Check sheet for the drawn part. Datum: minimum x, y, z corner. Units: mm. A direction names the side the tool comes from. Round coordinates to 2 decimals unless told otherwise and drop trailing zeros. Write each loop counter-clockwise with the first axis right and the second up, starting at its lowest first coordinate (ties: lowest second). Pieces come first, ordered by that corner, then holes. Notation, with made-up numbers: (27.5, -34.5) - (53.5, -34.5) arc R12 ccw to (53.5, -27.5) - close; hole circle Ø5 at (35, 13.5). An arc over 180 degrees is marked (long way). Answer as a JSON object with one key per item and string values.
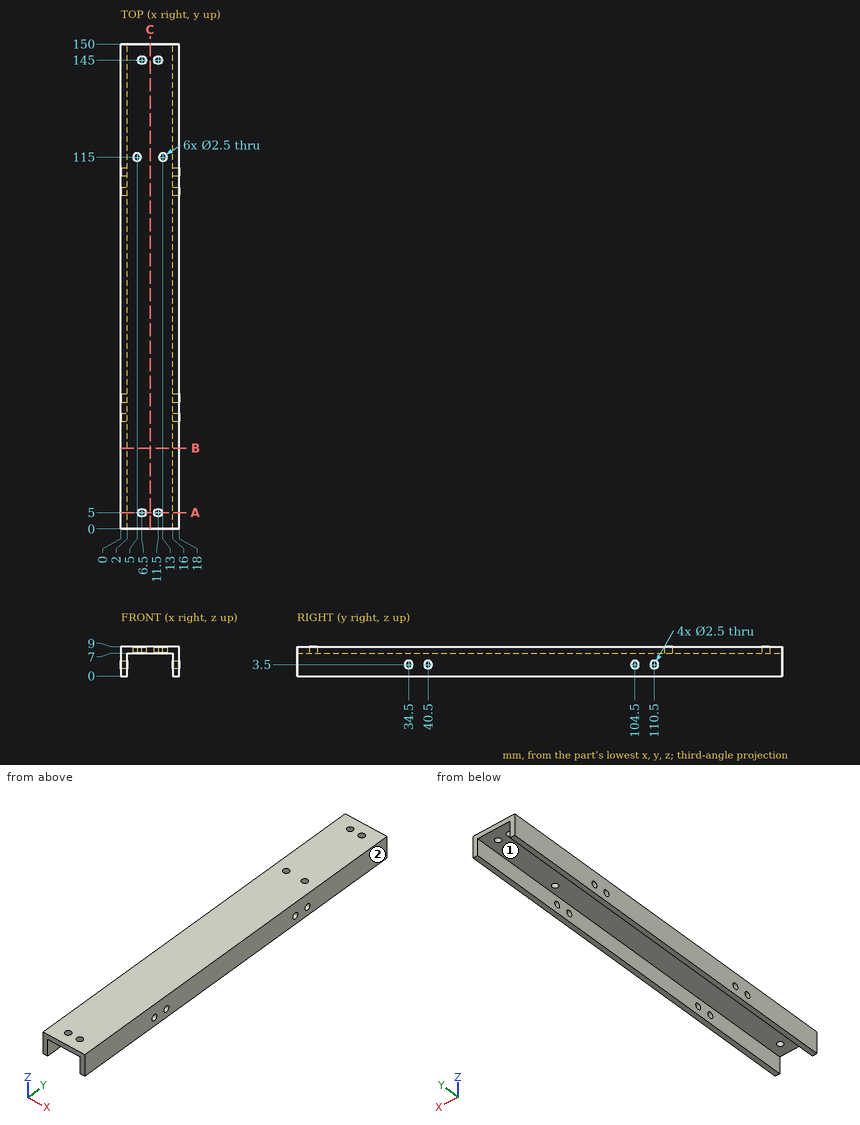
Q1. Set-up check for the marked faces 1 and 2: record each of +Z, -Z, +X, -X, +Y, -Y from which the full face is reachable in a straight line by a thin tool's end or side.
Geometry check:
{"face 1": "-Z, +Y, -Y", "face 2": "+Z, -Z, +X, +Y, -Y"}
Q2. Section check C-C, the plane x = 9. Record the cut outline in (y, z), then the cut area to 3 significant figures.
Geometry check:
{"outline": "(0, 7) - (150, 7) - (150, 9) - (0, 9) - close", "area": "300 mm2"}
Q3. Section check A-A, the plane y = 5. Record the cut outline in (x, z), then the cut area to 3 significant figures.
Geometry check:
{"outline": "(0, 0) - (2, 0) - (2, 7) - (5.25, 7) - (5.25, 9) - (0, 9) - close; (7.75, 7) - (10.25, 7) - (10.25, 9) - (7.75, 9) - close; (12.75, 7) - (16, 7) - (16, 0) - (18, 0) - (18, 9) - (12.75, 9) - close", "area": "54.0 mm2"}
Q4. Section check B-B, the plane y = 25. Record the cut outline in (x, z), then the cut area to 3 significant figures.
Geometry check:
{"outline": "(0, 0) - (2, 0) - (2, 7) - (16, 7) - (16, 0) - (18, 0) - (18, 9) - (0, 9) - close", "area": "64.0 mm2"}
Q5. Material ranges on line 1 along Y through (x, z) = (6.5, 7.65); line 2 along Y through (x, z) = (17.2, 3.5); line 3 along X through (y, z) = (115, 7.6), recorded low to high. Write a range as [from, to].
Geometry check:
{"line 1": "y = [0, 3.75], [6.25, 143.75], [146.25, 150]", "line 2": "y = [0, 33.25], [35.75, 39.25], [41.75, 103.25], [105.75, 109.25], [111.75, 150]", "line 3": "x = [0, 3.75], [6.25, 11.75], [14.25, 18]"}
Q6. Gauge pin test, flat ends, axial feed: P1, Ø2, axis at y = 40.5, z = 3.5, coming from the -X side; P2, Ø2, axis at x = 3.5, y = 110, coming from the -Z side. Record the tip position at first contact, or that the pin passes through.
Geometry check:
{"P1": "passes through", "P2": "stops at z = 7"}
